Source: CAD feature listing. Evaluate the final solid. Frame: model axes, mm. Face numbers are marked on the shaded views. A direction names the side the tool comes from. Round coordinates to 2 decimals unless told otherwise and drop trailing zeros. Order: outer loops, then holes, each group sorted by start corner. A loop starts at its lowest first (then second) coordinate and runs counter-clockwise, first axis right, second up. Notation, with made-up numbers: (78.5, 22) -> (83.5, 22) arc R28 ccw to (83.5, 53) -> close; hole circle Ø9 at (65.25, -38.5). An arc over 180 degrees is marked (long way). One line per item, written item: value. Start each with the question number.
1) Ray query, L1, parallel to Z at x = 5.75, y = -0.25; L2, parallel to Z at x = 5.75, y = 7.75; L3, parallel to X at y = -4, z = -16.5. Return the intervals inside material, ascending.
2) Section A-A (x = 0). Return the cut outline in (y, z), and give its area (3 significant figures).
3) Section C-C (z = -11). Return the cut outline in (x, y), and give its area (3 significant figures).
4) Section D-D (z = -1.25). Return the cut outline in (x, y).
5) Reachability of the marked faces 1 and 2 from +Z, -Z, +X, -X, +Y, -Y: full face, straight path, thin tool, end or side. Return the list, or none.
6) Pin query (flat end, axial travel): P1, Ø3, axis at x = -4, z = -6.5, coming from the -Y side; P2, Ø0.6, axis at x = -3.5, z = -1.5, coming from the +Y side; P3, Ø0.6, axis at x = 4.5, z = -0.5, coming from the -Y side. Return the tip coordinate at first contact, or that it passes through.
7) Section B-B (y = 0). Return the cut outline in (x, z), and give its area (3 significant figures).
```python
from build123d import *

# Parameters (mm, degrees)
F2_W     = 30
F2_H     = 3.5
F3_DEPTH = 2


with BuildPart() as f1:
    # F0 (on Front) → F1 (revolve)
    with BuildSketch(Plane.XZ):
        Polygon((12.5, 0), (0, 0), (0, -21), (8, -21), (8, -20), (10, -20), (10, -2.5), align=None)
    revolve(axis=Axis((0, 0, -12.648922), (0, 0, -1)))

    # F2 (on face) → F3 (cut)
    with BuildSketch(Plane.XY):
        with Locations((1.177149, 0)):
            Rectangle(F2_W, F2_H)
    extrude(amount=-F3_DEPTH, mode=Mode.SUBTRACT)


solid = f1.part
```
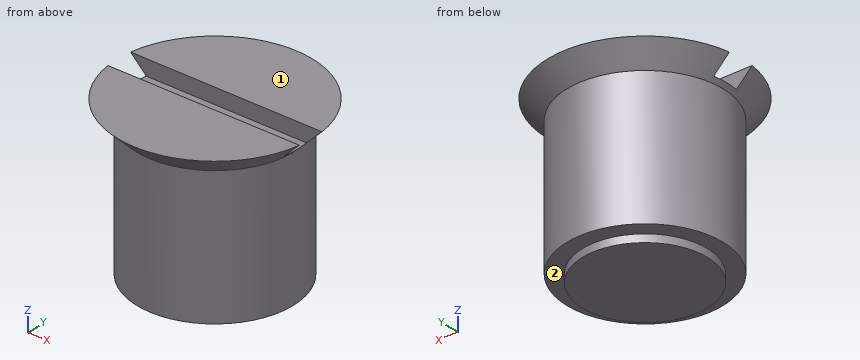
Findings:
1. L1: -21 to -2
1. L2: -20 to 0
1. L3: -9.17 to 9.17
2. outline: (-12.5, 0) -> (-10, -2.5) -> (-10, -20) -> (-8, -20) -> (-8, -21) -> (8, -21) -> (8, -20) -> (10, -20) -> (10, -2.5) -> (12.5, 0) -> (1.75, 0) -> (1.75, -2) -> (-1.75, -2) -> (-1.75, 0) -> close
2. area: 415 mm2
3. outline: circle Ø20 at (0, 0)
3. area: 314 mm2
4. outline: (-11.11, -1.75) arc R11.25 ccw to (11.11, -1.75) -> close; (-11.11, 1.75) -> (11.11, 1.75) arc R11.25 ccw to start
5. face 1: +Z, +X, -X, +Y, -Y
5. face 2: -Z
6. P1: y = -9.68
6. P2: y = 10.76
6. P3: y = -11.47
7. outline: (-10.5, -2) -> (-10, -2.5) -> (-10, -20) -> (-8, -20) -> (-8, -21) -> (8, -21) -> (8, -20) -> (10, -20) -> (10, -2.5) -> (10.5, -2) -> close
7. area: 376 mm2
